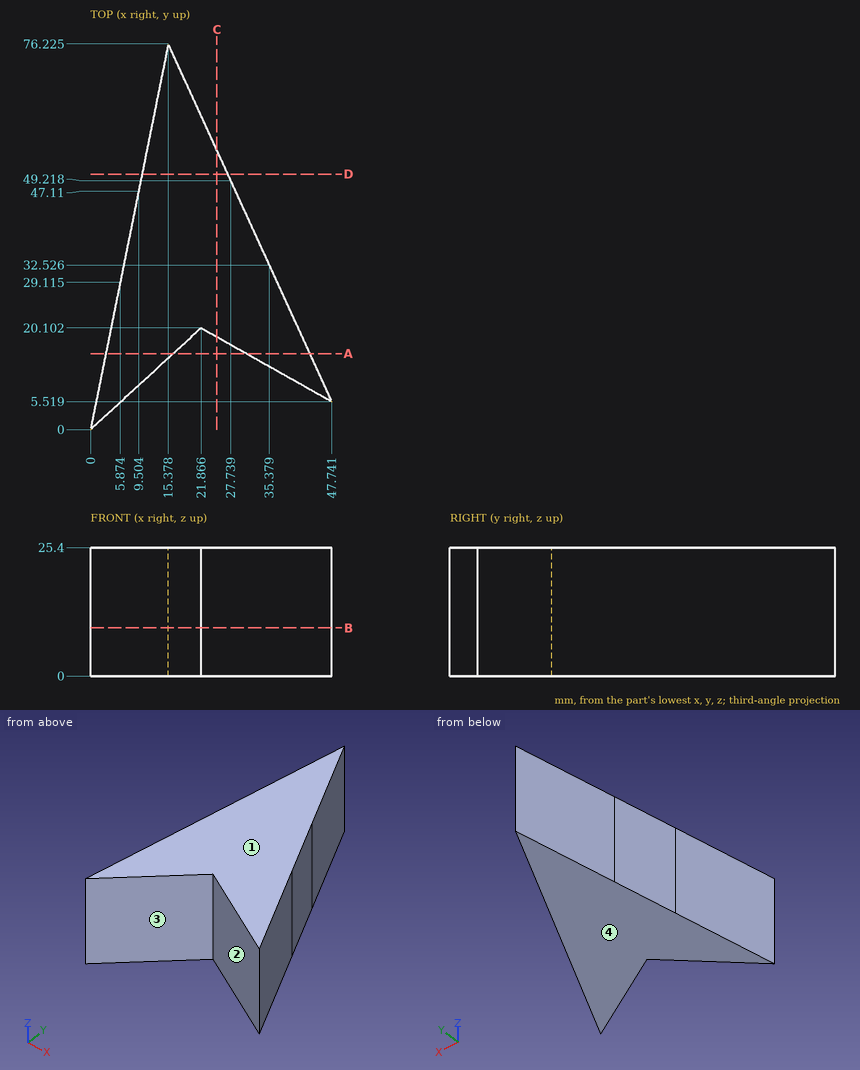
Could you check a few things on this drawing? It's one solid part, dimensions in mm from its lowest x, y, z. A direction names the side the tool comes from. Give positions to 0.01 mm unless a question says otherwise; leave off trailing zeros. Order: outer loops, then holes, each group sorted by start corner. A loop starts at its lowest first (then second) coordinate and runs counter-clockwise, first axis right, second up. Notation, with made-up numbers: (-34, -19) -> (-5, -19) arc R21 cw to (-5, 1) -> close; hole circle Ø10 at (-25, 44). An arc over 180 degrees is marked (long way). Use CSV: the item, a comma, the result in double quotes. Start each with the question number.
Item 1: Suppose I cut it at A-A (y = 15). List the corners of the cut face in (x, z) for me (1 decimal).
Item 2: Suppose I cut it at D-D (y = 50.5). List the corners of the cut face in (x, z) for me, and give its area (3 significant figures).
Item 3: If I drill on probe 1 along X at (y, z) = (13, 11) (1 decimal); probe 2 along X at (y, z) = (11.5, 4) (1 decimal); probe 3 along X at (y, z) = (28.5, 1.5), over which ranges is the centre line in solid material (lowest first)? Write a range as [from, to].
Item 4: I'm going to push flat-ended pins straight in: P1, Ø1, axis at x = 22, z = 22.5, coming from the -Y side (1 decimal); P2, Ø5, axis at x = 13, z = 4, coming from the -Y side; P3, Ø1, axis at x = 35, z = 16.5, coming from the -Y side. Where does each tip first touch, or does it pass through?
Item 5: Thinking about a two-plate mould opening in X: for the marked faces 3 and 4, which applies, pulls with the +X half, pulls with the -X half, needs draft (parallel to the pull), parting line crosses it, or undercut?
Item 6: Suppose I cut it at C-C (x = 25). List the corners of the cut face in (y, z) for me (1 decimal).
Item 7: On a 3-axis mill with a long thin cutter (end or side, diameter ignored), from which of +Z, -Z, +X, -X, +Y, -Y can I reach the whole of each face in a straight line? I mean the marked faces 1 and 2. Say none if no direction works.
Item 8: Suppose I cut it at B-B (z = 9.5). List the corners of the cut face in (x, y) for me (1 decimal).
Answer block:
1,outline,"(3, 0) -> (16.3, 0) -> (16.3, 25.4) -> (3, 25.4) -> close; (30.9, 0) -> (43.4, 0) -> (43.4, 25.4) -> (30.9, 25.4) -> close"
2,outline,"(10.19, 0) -> (27.15, 0) -> (27.15, 25.4) -> (10.19, 25.4) -> close"
2,area,"431 mm^2"
3,probe 1,"x = [2.6, 14.1], [34.5, 44.3]"
3,probe 2,"x = [2.3, 12.5], [37.1, 45]"
3,probe 3,"x = [5.75, 37.22]"
4,P1,"stops at y = 19.7"
4,P2,"stops at y = 9.65"
4,P3,"stops at y = 12.42"
5,face 3,"undercut"
5,face 4,"needs draft"
6,outline,"(18.3, 0) -> (55.2, 0) -> (55.2, 25.4) -> (18.3, 25.4) -> close"
7,face 1,"+Z, +X, -X, +Y, -Y"
7,face 2,"+Z, -Z, -Y"
8,outline,"(0, 0) -> (21.9, 20.1) -> (47.7, 5.5) -> (15.4, 76.2) -> close"
